from build123d import *

# Parameters (mm, degrees)
F1_DEPTH = 1.27
F2_R     = 2.54
F3_DEPTH = 25.4
F4_R     = 1.26999
F5_W     = 11.176
F5_H     = 8.128
F6_DEPTH = 0.7112


# Not quite as in the source:
# - a fillet or chamfer is up to 0.001 mm smaller than in the source, because OpenCascade refuses the exact size


with BuildPart() as f1:
    # F0 (on Front) → F1 (new body, symmetric)
    with BuildSketch(Plane.XZ):
        with BuildLine():
            ThreePointArc((-23.6793548387, -6.2969165191), (-18.6695586883, -4.7710273121), (-16.51, 0))
            ThreePointArc((-16.51, 0), (-18.6695586883, 4.7710273121), (-23.6793548387, 6.2969165191))
            ThreePointArc((-23.6793548387, 6.2969165191), (-29.21, 0), (-23.6793548387, -6.2969165191))
        make_face()
        with BuildLine():
            ThreePointArc((-23.6793548387, 6.2969165191), (-18.6695586883, 4.7710273121), (-16.51, 0))
            ThreePointArc((-16.51, 0), (-18.6695586883, -4.7710273121), (-23.6793548387, -6.2969165191))
            Line((-23.6793548387, -6.2969165191), (15.0351612903, -11.3344497343))
            ThreePointArc((15.0351612903, -11.3344497343), (5.08, 0), (15.0351612903, 11.3344497343))
            Line((15.0351612903, 11.3344497343), (-23.6793548387, 6.2969165191))
        make_face()
        with BuildLine():
            ThreePointArc((27.94, 0), (24.0527943611, 8.5878491618), (15.0351612903, 11.3344497343))
            ThreePointArc((15.0351612903, 11.3344497343), (5.08, 0), (15.0351612903, -11.3344497343))
            ThreePointArc((15.0351612903, -11.3344497343), (24.0527943611, -8.5878491618), (27.94, 0))
        make_face()
    extrude(amount=F1_DEPTH, both=True)

    # F2 (on face) → F3 (cut, symmetric)
    with BuildSketch(Plane.XZ.offset(1.27)):
        with Locations((-22.86, 0)):
            Circle(F2_R)
    extrude(amount=F3_DEPTH, both=True, mode=Mode.SUBTRACT)

    # F4 (radius 1.27 in the source; OpenCascade refuses exactly that, so slightly less here)
    f4_edges = [f1.edges().sort_by_distance(p)[0] for p in [
        (-4.322097, -1.27, 8.815683),
        (-4.322097, 1.27, 8.815683),
        (27.94, -1.27, 0),
        (15.035161, 0, -11.33445),
        (27.94, 1.27, 0),
        (15.035161, 0, 11.33445),
        (-29.21, -1.27, 0),
        (-25.4, 1.27, 0),
        (-25.4, -1.27, 0),
        (-29.21, 1.27, 0),
    ]]
    fillet(f4_edges, radius=F4_R)

    # F5 (on face) → F6 (cut)
    with BuildSketch(Plane.XZ.offset(1.27)):
        with Locations((12.192, -0.0039664305)):
            Rectangle(F5_W, F5_H)
    extrude(amount=-F6_DEPTH, mode=Mode.SUBTRACT)


solid = f1.part
Design review of the part built by this model. Coordinates are the model's own, in mm. Give positions to 0.01 mm unless a question says otherwise; leave off trailing zeros. Write item = value, one per line.
1) Clearance check with flat-ended pins moving along their axes: pin 1 Ø2.5 at (x, z) = (14, 0.5) entering from -Y; pin 2 Ø8 at (x, z) = (-22.86, 0) entering from +Y; pin 3 Ø1 at (x, y) = (-14.5, 0.5) entering from -Z; pin 4 Ø1 at (x, y) = (8, -0.5) entering from -Z. State where each tip first meets the part, or that it passes through.
Result sheet:
pin_1 = -0.56
pin_2 = 1.27
pin_3 = -7.53
pin_4 = -10.46
2) Draft analysis for pull direction Z (two halves, no side actions). For faces 1 (the face through (12, -0.559, 0)), 2 (the face through (5, -1.27, 0)), 3 (the face through (-4, 0.91, -8.47)), state which applies: +Z half, -Z half, draft (parallel to the pull), parting line (faces both ways), or undercut.
Result sheet:
face_1 = undercut
face_2 = draft
face_3 = -Z half
3) To check wall thickness, follow line 1 (X direction, y = -1.05, z = 1.75); line 2 (Y direction, x = 15, z = 0.75); line 3 (Z direction, x = -22.86, y = 0). State the ranges of each line that lie inside material, in increasing order.
Result sheet:
line_1 = -28.38 to -25.41, -20.31 to 6.6, 17.78 to 27.24
line_2 = -0.56 to 1.27
line_3 = -6.4 to -2.54, 2.54 to 6.4
